Source: CAD feature listing. Evaluate the final solid. Frame: model axes, mm. A direction names the side the tool comes from. Give positions to 0.01 mm unless a question says otherwise; leave off trailing zeros. Loops run counter-clockwise (first coordinate to the right, second up) from the corner with the lowest first, then second, coordinate; pieces in that order, holes last.
from build123d import *

# Parameters (mm, degrees)
SKETCH1_W           = 30
SKETCH1_H           = 40
BOSS_EXTRUDE1_DEPTH = 4
SKETCH2_W           = 18
SKETCH2_H           = 18
BOSS_EXTRUDE2_DEPTH = 40
SKETCH3_R           = 1.7
CUT_EXTRUDE1_DEPTH  = 53.017041145


with BuildPart() as part:
    # Sketch1 → Boss-Extrude1 (new body)
    with BuildSketch(Plane(origin=(0, 0, 0), x_dir=(0, 0, -1), z_dir=(1, 0, 0))):
        with Locations((4.583333333, -6.875)):
            Rectangle(SKETCH1_W, SKETCH1_H)
    extrude(amount=BOSS_EXTRUDE1_DEPTH)

    # Sketch2 → Boss-Extrude2 (add)
    with BuildSketch(Plane(origin=(4, 0, 0), x_dir=(0, 0, -1), z_dir=(1, 0, 0))):
        with Locations((4.583333333, 2.125)):
            Rectangle(SKETCH2_W, SKETCH2_H)
    extrude(amount=BOSS_EXTRUDE2_DEPTH)

    # Sketch3 → Cut-Extrude1 (cut, through all)
    with BuildSketch(Plane(origin=(4, 0, 0), x_dir=(0, 0, -1), z_dir=(1, 0, 0))):
        with Locations((-7.416666667, 3.125)):
            Circle(SKETCH3_R)
        with Locations((16.583333333, 3.125)):
            Circle(SKETCH3_R)
    extrude(amount=-CUT_EXTRUDE1_DEPTH, mode=Mode.SUBTRACT)


solid = part.part
1) Cut plane C-C (z = 6.25). Return loops of the section in (x, y) (3 decimals).
Checks:
outline: (0, -26.875) - (4, -26.875) - (4, 1.889) - (0, 1.889) - close; (0, 4.361) - (4, 4.361) - (4, 13.125) - (0, 13.125) - close
2) Contact query for flat-ended pins moving along their axis: P1, Ø6, axis at x = 28.5, z = -12, coming from the -Y side (3 decimals); P2, Ø6, axis at y = -14.5, z = 6.5, coming from the +X side; P3, Ø5.5, axis at x = 19, y = 6.5, coming from the -Z side; P4, Ø2, axis at y = 3.12, z = -16.58, coming from the +X side. Output: stop coordinate, or through.
Checks:
P1: stops at y = -6.875
P2: stops at x = 4
P3: stops at z = -13.58
P4: passes through
3) Pull-direction query (Y, two-part tool) for faces 4 (the flat face through (24, 11.125, -4)), 5 (the cylindrical face through (2.028, 3.636, 5.795)), 6 (the flat face through (24, 2, 4.417)), 7 (the cylindrical face through (2.028, 3.2, -14.885)); classes: released by +Y, released by -Y, zero draft, split by the parting line, or undercut.
Checks:
face 4: released by +Y
face 5: undercut
face 6: zero draft
face 7: undercut
4) Ray query, probe 1 along X at (y, z) = (-15, -7.75); probe 2 along Y at (x, z) = (15, -6) (3 decimals); probe 3 along Z at (x, y) = (16.5, 0). Return the intervals inside material, ascending.
Checks:
probe 1: x = 0 to 4
probe 2: y = -6.875 to 11.125
probe 3: z = -13.58 to 4.42
5) Reachability of faces 1 (the flat face through (2, -7, -19.583)), 2 (the flat face through (24, -6.875, -4)), 3 (the flat face through (24, 2, -13.583)) from +Z, -Z, +X, -X, +Y, -Y: full face, straight path, thin tool, end or side. Return the list, or none.
Checks:
face 1: -Z, +X, -X, +Y, -Y
face 2: +Z, -Z, +X, -Y
face 3: -Z, +X, +Y, -Y
6) Cut plane A-A (y = -3). Return loops of the section in (x, z), and give its area (3 significant figures).
Checks:
outline: (0, -19.58) - (4, -19.58) - (4, -13.58) - (44, -13.58) - (44, 4.42) - (4, 4.42) - (4, 10.42) - (0, 10.42) - close
area: 840 mm2
7) Cut plane B-B (z = -8.75). Return loops of the section in (x, y) (3 decimals).
Checks:
outline: (0, -26.875) - (4, -26.875) - (4, -6.875) - (44, -6.875) - (44, 11.125) - (4, 11.125) - (4, 13.125) - (0, 13.125) - close
8) Cut plane D-D (x = 3). Return loops of the section in (y, z) (3 decimals).
Checks:
outline: (-26.875, -19.583) - (13.125, -19.583) - (13.125, 10.417) - (-26.875, 10.417) - close; hole circle Ø3.4 at (3.125, -16.583); hole circle Ø3.4 at (3.125, 7.417)
